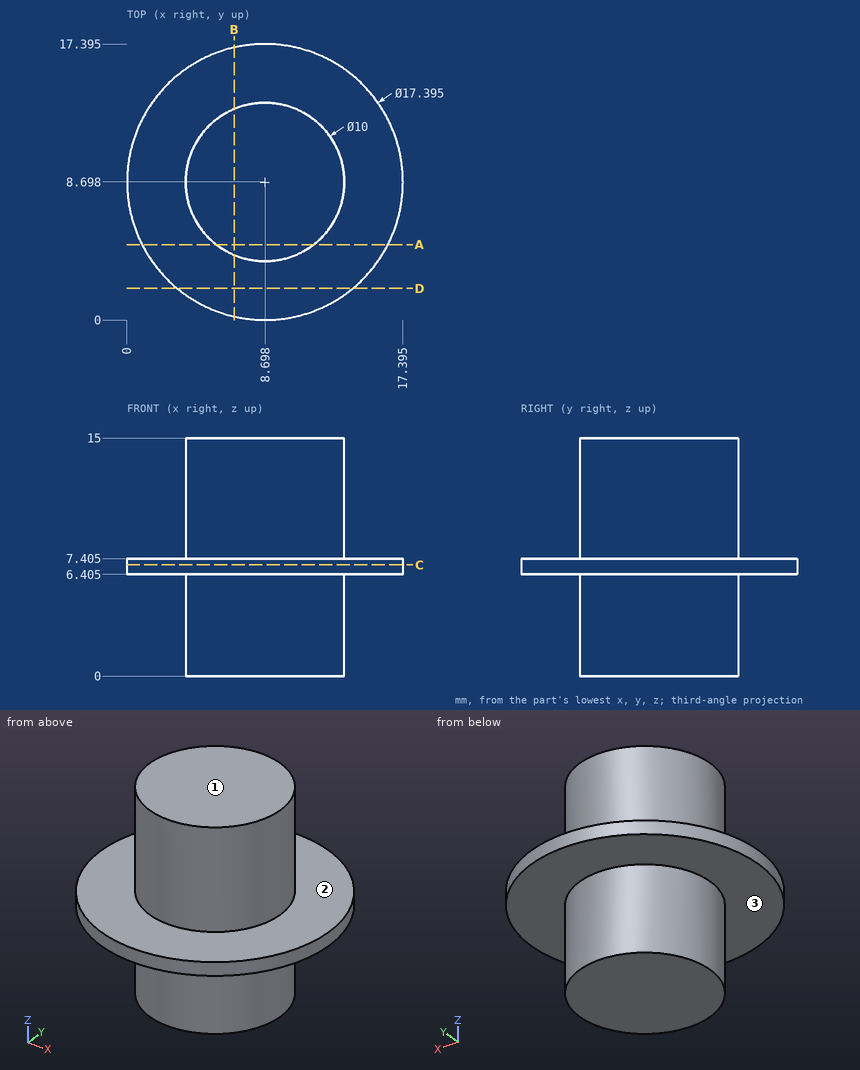
Source: three-view drawing plus pictorial views. Frame: mm from the lowest corner of the part. A direction names the side the tool comes from. Coordinates: 2 decimals unless noted, no trailing zeros. Loops run counter-clockwise (first coordinate to the right, second up) from the corner with the lowest first, then second, coordinate; pieces in that order, holes last. Notation, with made-up numbers: (13, 41.5) -> (24, 41.5) arc R34 ccw to (24, 80.5) -> close; hole circle Ø4 at (62, 56). An arc over 180 degrees is marked (long way). Answer in a Markdown table with one row per item. Add a question column.
Q1. Reachability of the marked faces 1, 2 and 3 from +Z, -Z, +X, -X, +Y, -Y: full face, straight path, thin tool, end or side. Return the list, or none.
Q2. Section A-A on y = 4.75. Return the cut outline in (x, z) (1 decimal).
Q3. Contact query for flat-ended pins moving along their axis: pin 1 Ø1 at (x, z) = (3.5, 6) entering from +Y; pin 2 Ø8 at (y, z) = (4, 9) entering from +X; pin 3 Ø3 at (x, z) = (13, 12) entering from -Y; pin 4 Ø1.5 at (y, z) = (15.5, 4) entering from -X. Output: stop coordinate, or through.
Q4. Section D-D on y = 2. Return the cut outline in (x, z) (1 decimal).
Q5. Ray query, line 1 along Z through (x, y) = (4, 2.5) (1 decimal); line 2 along X through (y, z) = (6.75, 4); line 3 along X through (y, z) = (4.25, 11.25) (1 decimal). Return the intervals inside material, ascending.
Q6. Section B-B on x = 6.75. Return the cut outline in (y, z) (1 decimal), and give its area (3 significant figures).
Q7. Section C-C on z = 7. Return the cut outline in (x, y) (1 decimal), and give its area (3 significant figures).
Computed values:
| question | item | result |
|---|---|---|
| 1 | face 1 | +Z, +X, -X, +Y, -Y |
| 1 | face 2 | +Z |
| 1 | face 3 | -Z |
| 2 | outline | (0.9, 6.4) -> (5.6, 6.4) -> (5.6, 0) -> (11.8, 0) -> (11.8, 6.4) -> (16.4, 6.4) -> (16.4, 7.4) -> (11.8, 7.4) -> (11.8, 15) -> (5.6, 15) -> (5.6, 7.4) -> (0.9, 7.4) -> close |
| 3 | pin 1 | stops at y = 15.88 |
| 3 | pin 2 | stops at x = 17.33 |
| 3 | pin 3 | stops at y = 4.56 |
| 3 | pin 4 | passes through |
| 4 | outline | (3.1, 6.4) -> (14.2, 6.4) -> (14.2, 7.4) -> (3.1, 7.4) -> close |
| 5 | line 1 | z = 6.4 to 7.4 |
| 5 | line 2 | x = 4.09 to 13.3 |
| 5 | line 3 | x = 6.4 to 11 |
| 6 | outline | (0.2, 6.4) -> (4.1, 6.4) -> (4.1, 0) -> (13.3, 0) -> (13.3, 6.4) -> (17.2, 6.4) -> (17.2, 7.4) -> (13.3, 7.4) -> (13.3, 15) -> (4.1, 15) -> (4.1, 7.4) -> (0.2, 7.4) -> close |
| 6 | area | 146 mm^2 |
| 7 | outline | circle Ø17.4 at (8.7, 8.7) |
| 7 | area | 238 mm^2 |
